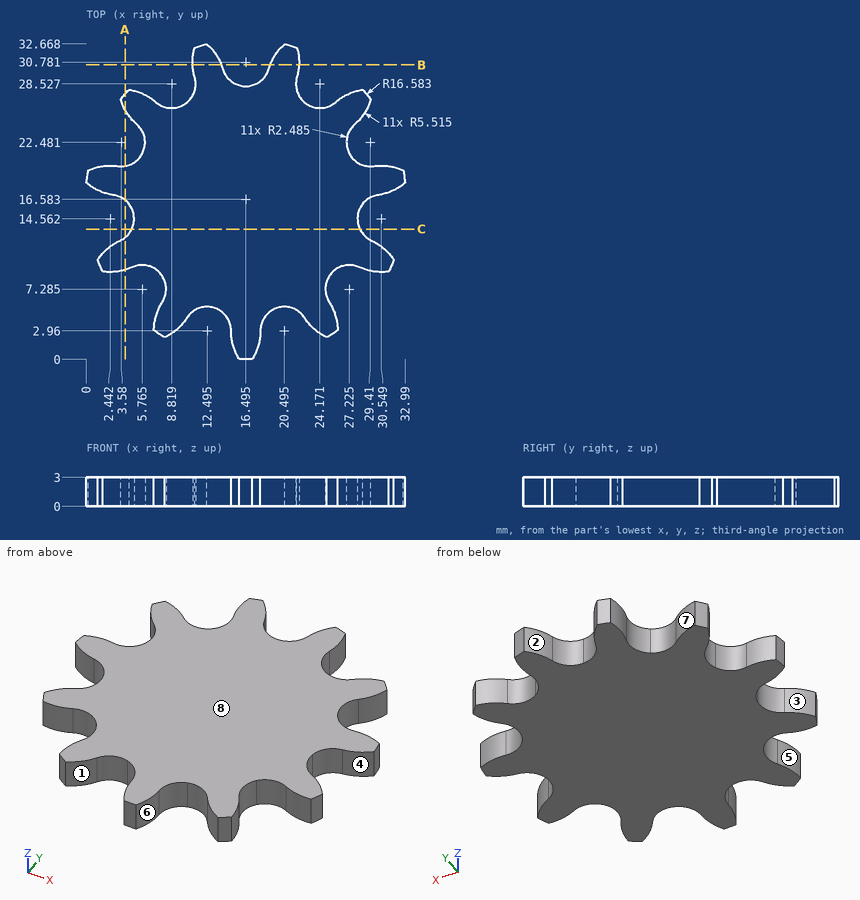
Geometry: see drawing. Coordinates: mm, zero at the bounding-box minimum. A direction names the side the tool comes from. Coordinates: 2 decimals unless noted, no trailing zeros. Order: outer loops, then holes, each group sorted by start corner. A loop starts at its lowest first (then second) coordinate and runs counter-clockwise, first axis right, second up. Notation, with made-up numbers: M 68.5,-23 L 73.5,-23 A9 cw 73.5,-6 Z; hole C -6.5,79.25 d5. An arc over 180 degrees is marked long. Answer in a Markdown table with one row per item. Add a question column.
Q1. Reachability of the marked faces 4, 5, 6, 7 and 8 from +Z, -Z, +X, -X, +Y, -Y: full face, straight path, thin tool, end or side. Return the list, or none.
Q2. Section query A-A on x = 4. Return the cut outline in (y, z) (1 decimal).
Q3. Mould query, pull axis Y, two halves, no side actions, for the marked faces 1, 2 and 3. Classes: released by +Y, released by -Y, zero draft, split by the parting line, or undercut.
Q4. Line query: L1, parallel to X at y = 5, z = 0.35 (1 decimal); L2, parallel to X at y = 3.5, z = 1.25 (1 decimal); L3, parallel to Y at x = 8, z = 2.5 (1 decimal). Output: solid intervals per line, ascending.
Q5. Section query C-C on y = 13.5. Return the cut outline in (x, z).
Q6. Section query B-B on y = 30.5. Return the cut outline in (x, z).
Completed:
| question | item | result |
|---|---|---|
| 1 | face 4 | +Z, -Z, +X |
| 1 | face 5 | +Z, -Z, -X |
| 1 | face 6 | +Z, -Z, -Y |
| 1 | face 7 | +Z, -Z, +Y |
| 1 | face 8 | +Z, +X, -X, +Y, -Y |
| 2 | outline | M 9.3,0 L 12.6,0 L 12.6,3 L 9.3,3 Z; M 16.5,0 L 20,0 L 20,3 L 16.5,3 Z; M 25.8,0 L 27.5,0 L 27.5,3 L 25.8,3 Z |
| 3 | face 1 | released by -Y |
| 3 | face 2 | released by +Y |
| 3 | face 3 | undercut |
| 4 | L1 | x = 7.4 to 11.1, 13.9 to 19.1, 21.9 to 25.6 |
| 4 | L2 | x = 7 to 9.8, 14.9 to 18.1, 23.2 to 26 |
| 4 | L3 | y = 2.3 to 6.2, 8.4 to 26.2 |
| 5 | outline | M 4.69,0 L 28.3,0 L 28.3,3 L 4.69,3 Z |
| 6 | outline | M 10.99,0 L 13.97,0 L 13.97,3 L 10.99,3 Z; M 19.02,0 L 22,0 L 22,3 L 19.02,3 Z |
